Part model, mm, in its own coordinate system. Face numbers are marked on the shaded views. Give positions to 0.01 mm unless a question says otherwise; leave off trailing zeros. Order: outer loops, then holes, each group sorted by start corner. A loop starts at its lowest first (then second) coordinate and runs counter-clockwise, first axis right, second up. Notation, with made-up numbers: (50.5, 52.5) - (55.5, 52.5) arc R19 ccw to (55.5, 66.5) - close; hole circle Ø7 at (-15, 5.25). An arc over 180 degrees is marked (long way). One line per item, written item: value.
```python
from build123d import *

# Parameters (mm, degrees)
SKETCH1_W           = 80
SKETCH1_H           = 80
SKETCH1_R           = 36
SKETCH1_R_2         = 34
BOSS_EXTRUDE3_DEPTH = 2
BOSS_EXTRUDE4_START = 110
SKETCH1_7_R         = 36
SKETCH1_7_R_2       = 34
BOSS_EXTRUDE4_DEPTH = 110
BOSS_EXTRUDE5_DEPTH = 77.35


with BuildPart() as part:
    # Sketch1 → Boss-Extrude3 (new body)
    # profile 1 of 2: a face of its own
    with BuildSketch(Plane(origin=(0, 0, 0), x_dir=(1, 0, 0), z_dir=(0, 1, 0))):
        Rectangle(SKETCH1_W, SKETCH1_H)
        Circle(SKETCH1_R, mode=Mode.SUBTRACT)
    # profile 2 of 2: a face of its own
    with BuildSketch(Plane(origin=(0, 0, 0), x_dir=(1, 0, 0), z_dir=(0, 1, 0))):
        Circle(SKETCH1_R)
        with Locations(Location((0, 0, 0), (0, 0, 270))):
            Circle(SKETCH1_R_2, mode=Mode.SUBTRACT)
    extrude(amount=-BOSS_EXTRUDE3_DEPTH)

    # Sketch1<7> → Boss-Extrude4 (add)
    with BuildSketch(Plane(origin=(0, 0, 0), x_dir=(1, 0, 0), z_dir=(0, 1, 0)).offset(BOSS_EXTRUDE4_START)):
        with Locations(Location((0, 0, 0), (0, 0, 270))):
            Circle(SKETCH1_7_R)
        with Locations(Location((0, 0, 0), (0, 0, 270))):
            Circle(SKETCH1_7_R_2, mode=Mode.SUBTRACT)
    extrude(amount=-BOSS_EXTRUDE4_DEPTH)

    # Sketch3 → Boss-Extrude5 (add)
    with BuildSketch(Plane.XY.offset(40)):
        Polygon((-32.3, -2), (-34.8, -2), (-34.8, -4.3), (-37.3, -4.3), (-37.3, -6.3), (-32.3, -6.3), align=None)
        Polygon((32.3, -6.3), (37.3, -6.3), (37.3, -4.3), (34.8, -4.3), (34.8, -2), (32.3, -2), align=None)
    extrude(amount=-BOSS_EXTRUDE5_DEPTH)


solid = part.part
```
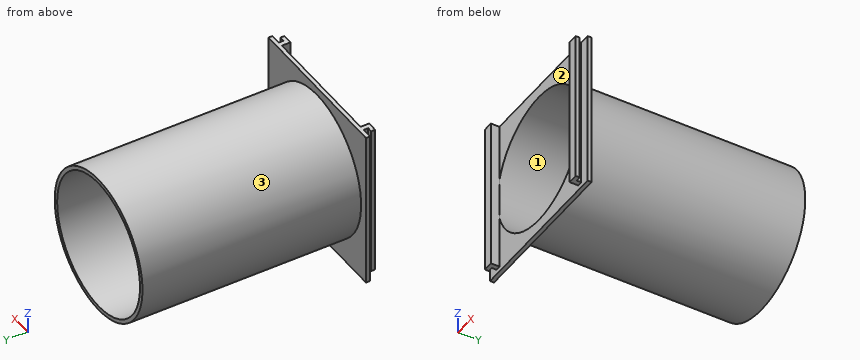
1) Two-plate mould, pull along Z, no slides. Class the marked faces 1, 2 and 3: pulls with the +Z half, pulls with the -Z half, needs draft (parallel to the pull), parting line crosses it, or undercut.
Answer:
face 1: undercut
face 2: needs draft
face 3: parting line crosses it
2) Drop flat-ended pins along their axis: P1, Ø2, axis at x = 17.5, y = 18, coming from the +Z side; P2, Ø3.5, axis at y = -5, z = -15.5, coming from the +X side; P3, Ø0.5, axis at x = 33, z = 0, coming from the +Y side; P4, Ø2.5, axis at y = -3, z = -17.5, coming from the +X side. Give the stop position or say it passes through.
Answer:
P1: stops at z = 32
P2: stops at x = 37.3
P3: stops at y = -2
P4: stops at x = 40
3) Wall check: line 1 along X through (y, z) = (24, 0); line 2 along X through (y, z) = (48.5, -21); line 3 along Y through (x, z) = (-14.5, -31). Give the ranges that are in metal, low to high. Write a range as [from, to].
Answer:
line 1: x = [-36, -34], [34, 36]
line 2: x = [-29.24, -26.74], [26.74, 29.24]
line 3: y = [-2, 110]
4) Slice it at A-A on x = 0. Write the cut outline in (y, z), then the cut area to 3 significant figures.
Answer:
outline: (-2, -40) - (0, -40) - (0, -36) - (110, -36) - (110, -34) - (-2, -34) - close; (-2, 34) - (110, 34) - (110, 36) - (0, 36) - (0, 40) - (-2, 40) - close
area: 464 mm2
5) Slice it at B-B on z = 0. Write the cut outline in (x, y).
Answer:
outline: (-40, -2) - (-34.8, -2) - (-34.8, -4.3) - (-37.3, -4.3) - (-37.3, -6.3) - (-32.3, -6.3) - (-32.3, -2) - (-34, -2) - (-34, 110) - (-36, 110) - (-36, 0) - (-40, 0) - close; (32.3, -6.3) - (37.3, -6.3) - (37.3, -4.3) - (34.8, -4.3) - (34.8, -2) - (40, -2) - (40, 0) - (36, 0) - (36, 110) - (34, 110) - (34, -2) - (32.3, -2) - close
6) Slice it at D-D on z = -19. Write the cut outline in (x, y).
Answer:
outline: (-40, -2) - (-34.8, -2) - (-34.8, -4.3) - (-37.3, -4.3) - (-37.3, -6.3) - (-32.3, -6.3) - (-32.3, -2) - (-28.2, -2) - (-28.2, 110) - (-30.58, 110) - (-30.58, 0) - (-40, 0) - close; (28.2, -2) - (32.3, -2) - (32.3, -6.3) - (37.3, -6.3) - (37.3, -4.3) - (34.8, -4.3) - (34.8, -2) - (40, -2) - (40, 0) - (30.58, 0) - (30.58, 110) - (28.2, 110) - close
7) Slice it at C-C on y = 12.5. Write the cut outline in (x, z), then the cut area to 3 significant figures.
Answer:
outline: circle Ø72 at (0, 0); hole circle Ø68 at (0, 0)
area: 440 mm2
